Autodesk Inventor part; units mm, degrees
ref_plane "YZ Plane" through (0, 0, 0) normal (1, 0, 0) x (0, 1, 0)
ref_plane "XZ Plane" through (0, 0, 0) normal (0, 1, 0) x (-1, 0, 0)
ref_plane "XY Plane" through (0, 0, 0) normal (0, 0, 1) x (1, 0, 0)
sketch "Boceto1" plane through (0, 0, 0) normal (0, 1, 0) x (-1, 0, 0)
  circle A0 centre (0, 0) radius 10
  line L0 (10, 0) -> (3.0902, -9.5106)
  line L1 (3.0902, -9.5106) -> (-8.0902, -5.8779)
  line L2 (-8.0902, -5.8779) -> (-8.0902, 5.8779)
  line L3 (-8.0902, 5.8779) -> (3.0902, 9.5106)
  line L4 (3.0902, 9.5106) -> (10, 0)
  line L5 (-7.6902, -5.5872) -> (2.9374, -9.0403)
  line L6 (2.9374, -9.0403) -> (9.5056, 0)
  line L7 (9.5056, 0) -> (2.9374, 9.0403)
  line L8 (2.9374, 9.0403) -> (-7.6902, 5.5872)
  line L9 (-7.6902, 5.5872) -> (-7.6902, -5.5872)
  dimension "d0" = 20
  dimension "d1" = 0.4
extrude "Extrusión1" add sketch "Boceto1" along normal blind 1 contours L0 L1 L2 L3 L4
extrude "Extrusión2" add sketch "Boceto1" along normal blind 0.5 contours L9 L8 L7 L6 L5
sketch "Boceto2" plane through (0, 0.5, 0) normal (0, 1, 0) x (1, 0, 0)
  line L0 (8.0902, -5.8779) -> (8.0902, 5.8779)
  line L1 (8.0902, -5.8779) -> (3.9, 0)
  line L2 (3.9, 0) -> (8.0902, 5.8779)
  circle A0 centre (0, 0) radius 10
  line L3 (8.0902, 5.8779) -> (1.2052, 3.7091)
  line L4 (1.2052, 3.7091) -> (-3.0902, 9.5106)
  line L5 (-3.0902, 9.5106) -> (-3.1552, 2.2924)
  line L6 (-3.1552, 2.2924) -> (-10, 0)
  line L7 (-10, 0) -> (-3.1552, -2.2924)
  line L8 (-3.1552, -2.2924) -> (-3.0902, -9.5106)
  line L9 (-3.0902, -9.5106) -> (1.2052, -3.7091)
  line L10 (1.2052, -3.7091) -> (8.0902, -5.8779)
  dimension "d6" = 3.9
  dimension "d9" = 360
extrude "Extrusión3" add sketch "Boceto2" along normal blind 0.5 contours L10 L9 L8 L7 L6 L5 L4 L3 L2 L1
properties part number "Pieza de practica 1"
Verification items for the finished model (mm, model axes). A direction names the side the tool comes from. Round coordinates to 2 decimals unless told otherwise and drop trailing zeros. Loops run counter-clockwise (first coordinate to the right, second up) from the corner with the lowest first, then second, coordinate; pieces in that order, holes last. Notation, with made-up numbers: (89, 13.25) - (136, 13.25) arc R18 cw to (136, 37.25) - close; hole circle Ø5 at (38, -2.5). An arc over 180 degrees is marked (long way). Use a Markdown table: item, result. Add a question column.
1. Thickness scan on probe 1 along Z at (x, y) = (-5.5, 0.8); probe 2 along Z at (x, y) = (-4, 0.6); probe 3 along X at (y, z) = (0.6, -2.5). Record the ranges inside material, lowest first. Write a range as [from, to].
2. Section check A-A, the plane y = 0.85. Record the boundary of the cut face in (x, z).
3. Access from +Z, -Z, +X, -X, +Y, -Y to the whole of each face (thin tool, end or side, straight path). Record for faces 1 (the face through (-1, 0, 0)), 2 (the face through (6, 0.5, 0)).
4. Section check C-C, the plane x = 5.75. Record the boundary of the cut face in (y, z).
5. Release check for a two-part mould opening along X. For faces 3 (the face through (-1, 1, 0)), 4 (the face through (-6.5, 0.49, 4.82)), 5 (the face through (-5, 0.5, -4)) record: released by +X, released by -X, zero draft, split by the parting line, or undercut.
6. Section check B-B, the plane z = 3. Record the boundary of the cut face in (x, y), plus the area to 3 significant figures.
7. Gauge pin test, flat ends, axial feed: pin 1 (5 mm diameter, centred on x = 4, z = 4, fed in from -Y); pin 2 (0.6 mm diameter, centred on y = 1, z = -2.5, fed in from -X). Record the tip position at first contact, or that the pin passes through.
8. Section check D-D, the plane z = 7. Record the boundary of the cut face in (x, y).
Checks:
| question | item | result |
|---|---|---|
| 1 | probe 1 | z = [-6.19, -5.51], [-1.51, 1.51], [5.51, 6.19] |
| 1 | probe 2 | z = [-8.26, -7.58], [-2.01, 2.01], [7.58, 8.26] |
| 1 | probe 3 | x = [-8.18, -7.69], [-3.15, 5.68], [7.69, 8.09] |
| 2 | outline | (-10, 0) - (-3.09, -9.51) - (8.09, -5.88) - (8.09, 5.88) - (-3.09, 9.51) - close; hole (-9.35, -0.22) - (-3.1, -8.82) - (-3.16, -2.29) - close; hole (-9.35, 0.22) - (-3.16, 2.29) - (-3.1, 8.82) - close; hole (-2.68, -8.96) - (7.43, -5.67) - (1.21, -3.71) - close; hole (-2.68, 8.96) - (1.21, 3.71) - (7.43, 5.67) - close; hole (3.9, 0) - (7.69, -5.32) - (7.69, 5.32) - close |
| 3 | face 1 | +Z, -Z, +X, -X, -Y |
| 3 | face 2 | +Y |
| 4 | outline | (0, -6.64) - (1, -6.64) - (1, -6.22) - (0.5, -6.22) - (0.5, -5.14) - (1, -5.14) - (1, -2.6) - (0.5, -2.6) - (0.5, 2.6) - (1, 2.6) - (1, 5.14) - (0.5, 5.14) - (0.5, 6.22) - (1, 6.22) - (1, 6.64) - (0, 6.64) - close |
| 5 | face 3 | zero draft |
| 5 | face 4 | released by -X |
| 5 | face 5 | undercut |
| 6 | outline | (-7.82, 0) - (8.09, 0) - (8.09, 1) - (7.69, 1) - (7.69, 0.5) - (6.04, 0.5) - (6.04, 1) - (-3.15, 1) - (-3.15, 0.5) - (-7.33, 0.5) - (-7.33, 1) - (-7.82, 1) - close |
| 6 | area | 13.0 mm^2 |
| 7 | pin 1 | stops at y = 0 |
| 7 | pin 2 | stops at x = -8.4 |
| 8 | outline | (-4.91, 0) - (4.64, 0) - (4.64, 1) - (3.34, 1) - (3.34, 0.5) - (-1.23, 0.5) - (-1.23, 1) - (-3.11, 1) - (-3.11, 0.5) - (-4.42, 0.5) - (-4.42, 1) - (-4.91, 1) - close |
